from build123d import *

# Parameters (mm, degrees)
SKETCH1_W                    = 96
SKETCH1_H                    = 1
BASE_FLANGE1_DEPTH           = 329.72
EDGE_FLANGE1_STRIP_W         = 5.4732
EDGE_FLANGE1_STRIP_H         = 1
EDGE_FLANGE1_STRIP_CUT_DEPTH = 96
EDGE_FLANGE1_DEPTH           = 96
EDGE_FLANGE2_STRIP_W         = 5.4732
EDGE_FLANGE2_STRIP_H         = 1
EDGE_FLANGE2_STRIP_CUT_DEPTH = 96
EDGE_FLANGE2_DEPTH           = 96
EDGE_FLANGE3_STRIP_W         = 5.4732
EDGE_FLANGE3_STRIP_H         = 1
EDGE_FLANGE3_STRIP_CUT_DEPTH = 96
EDGE_FLANGE3_DEPTH           = 96
EDGE_FLANGE4_STRIP_W         = 5.4732
EDGE_FLANGE4_STRIP_H         = 1
EDGE_FLANGE4_STRIP_CUT_DEPTH = 96
EDGE_FLANGE4_DEPTH           = 96
CUT_EXTRUDE1_DEPTH           = 10
SKETCH23_R                   = 8
CUT_EXTRUDE4_DEPTH           = 10


# Sheet-metal steps are written as plain solids
with BuildPart() as part:
    # Sketch1 → Base-Flange1 (new body)
    with BuildSketch(Plane.XY):
        with Locations((48, -0.5)):
            Rectangle(SKETCH1_W, SKETCH1_H)
    extrude(amount=BASE_FLANGE1_DEPTH)

    # Edge-Flange1 strip (across the edge) → Edge-Flange1 strip cut (cut)
    with BuildSketch(Plane(origin=(0, 0, 329.72), x_dir=(0, 0, -1), z_dir=(1, 0, 0))):
        with Locations((-1, -0.5)):
            Rectangle(EDGE_FLANGE1_STRIP_W, EDGE_FLANGE1_STRIP_H)
    extrude(amount=EDGE_FLANGE1_STRIP_CUT_DEPTH, mode=Mode.SUBTRACT)

    # Edge-Flange1 section (across the edge) → Edge-Flange1 (add)
    with BuildSketch(Plane(origin=(0, 0, 329.72), x_dir=(0, 0, -1), z_dir=(1, 0, 0))):
        with BuildLine():
            Line((0, 0.7366), (0, 35))
            Line((0, 35), (1, 35))
            Line((1, 35), (1, 0.7366))
            ThreePointArc((1, 0.7366), (1.215745145, 0.215745145), (1.7366, 0))
            Line((1.7366, 0), (1.7366, -1))
            ThreePointArc((1.7366, -1), (0.508638364, -0.491361636), (0, 0.7366))
        make_face()
    extrude(amount=EDGE_FLANGE1_DEPTH)

    # Edge-Flange2 strip (across the edge) → Edge-Flange2 strip cut (cut)
    with BuildSketch(Plane.ZY.offset(-96)):
        with Locations((-1, -0.5)):
            Rectangle(EDGE_FLANGE2_STRIP_W, EDGE_FLANGE2_STRIP_H)
    extrude(amount=EDGE_FLANGE2_STRIP_CUT_DEPTH, mode=Mode.SUBTRACT)

    # Edge-Flange2 section (across the edge) → Edge-Flange2 (add)
    with BuildSketch(Plane.ZY.offset(-96)):
        with BuildLine():
            Line((0, 0.7366), (0, 35))
            Line((0, 35), (1, 35))
            Line((1, 35), (1, 0.7366))
            ThreePointArc((1, 0.7366), (1.215745145, 0.215745145), (1.7366, 0))
            Line((1.7366, 0), (1.7366, -1))
            ThreePointArc((1.7366, -1), (0.508638364, -0.491361636), (0, 0.7366))
        make_face()
    extrude(amount=EDGE_FLANGE2_DEPTH)

    # Edge-Flange3 strip (across the edge) → Edge-Flange3 strip cut (cut)
    with BuildSketch(Plane(origin=(0, 35, 328.72), x_dir=(0, -1, 0), z_dir=(1, 0, 0))):
        with Locations((-1, -0.5)):
            Rectangle(EDGE_FLANGE3_STRIP_W, EDGE_FLANGE3_STRIP_H)
    extrude(amount=EDGE_FLANGE3_STRIP_CUT_DEPTH, mode=Mode.SUBTRACT)

    # Edge-Flange3 section (across the edge) → Edge-Flange3 (add)
    with BuildSketch(Plane(origin=(0, 35, 328.72), x_dir=(0, -1, 0), z_dir=(1, 0, 0))):
        with BuildLine():
            Line((0, 0.7366), (0, 27))
            Line((0, 27), (1, 27))
            Line((1, 27), (1, 0.7366))
            ThreePointArc((1, 0.7366), (1.215745145, 0.215745145), (1.7366, 0))
            Line((1.7366, 0), (1.7366, -1))
            ThreePointArc((1.7366, -1), (0.508638364, -0.491361636), (0, 0.7366))
        make_face()
    extrude(amount=EDGE_FLANGE3_DEPTH)

    # Edge-Flange4 strip (across the edge) → Edge-Flange4 strip cut (cut)
    with BuildSketch(Plane(origin=(96, 35, 1), x_dir=(0, -1, 0), z_dir=(-1, 0, 0))):
        with Locations((-1, -0.5)):
            Rectangle(EDGE_FLANGE4_STRIP_W, EDGE_FLANGE4_STRIP_H)
    extrude(amount=EDGE_FLANGE4_STRIP_CUT_DEPTH, mode=Mode.SUBTRACT)

    # Edge-Flange4 section (across the edge) → Edge-Flange4 (add)
    with BuildSketch(Plane(origin=(96, 35, 1), x_dir=(0, -1, 0), z_dir=(-1, 0, 0))):
        with BuildLine():
            Line((0, 0.7366), (0, 27))
            Line((0, 27), (1, 27))
            Line((1, 27), (1, 0.7366))
            ThreePointArc((1, 0.7366), (1.215745145, 0.215745145), (1.7366, 0))
            Line((1.7366, 0), (1.7366, -1))
            ThreePointArc((1.7366, -1), (0.508638364, -0.491361636), (0, 0.7366))
        make_face()
    extrude(amount=EDGE_FLANGE4_DEPTH)

    # Sketch22 → Cut-Extrude1 (cut)
    with BuildSketch(Plane(origin=(0, 0, 0), x_dir=(1, 0, 0), z_dir=(0, 1, 0))):
        with BuildLine():
            Line((70, -214.9834), (70, -287.9834))
            ThreePointArc((70, -287.9834), (77, -294.9834), (84, -287.9834))
            Line((84, -287.9834), (84, -214.9834))
            ThreePointArc((84, -214.9834), (77, -207.9834), (70, -214.9834))
        make_face()
        with BuildLine():
            Line((70, -114.7366), (70, -41.7366))
            ThreePointArc((70, -41.7366), (77, -34.7366), (84, -41.7366))
            Line((84, -41.7366), (84, -114.7366))
            ThreePointArc((84, -114.7366), (77, -121.7366), (70, -114.7366))
        make_face()
    extrude(amount=-CUT_EXTRUDE1_DEPTH, mode=Mode.SUBTRACT)

    # Sketch23 → Cut-Extrude4 (cut)
    with BuildSketch(Plane(origin=(0, 0, 0), x_dir=(1, 0, 0), z_dir=(0, 1, 0))):
        with Locations(Location((25, -164.86, 0), (0, 0, 270))):
            Circle(SKETCH23_R)
    extrude(amount=-CUT_EXTRUDE4_DEPTH, mode=Mode.SUBTRACT)


solid = part.part
Input: part model. Units: mm. Frame: model coordinates. A direction names the side the tool comes from. Round coordinates to 2 decimals unless told otherwise and drop trailing zeros. Order: outer loops, then holes, each group sorted by start corner. A loop starts at its lowest first (then second) coordinate and runs counter-clockwise, first axis right, second up. Notation, with made-up numbers: (36.5, 7) - (46.5, 7) arc R22 ccw to (46.5, 26) - close; hole circle Ø9 at (60, 29.25). An arc over 180 degrees is marked (long way). Use a Markdown table: item, result.
1. Access query for faces 1 (the face through (47, 35, 315)), 2 (the face through (77.154, -0.493, 121.735)), 3 (the face through (47, 17, 328.72)). Directions: +Z, -Z, +X, -X, +Y, -Y. A direction counts if a zero-diameter tool reaches every point of the face in a straight line with its end or side. Return the directions, or none.
Evaluation:
| item | result |
|---|---|
| face 1 | +Z, -Z, +X, -X, +Y |
| face 2 | +Y, -Y |
| face 3 | +X, -X |
2. Section B-B on x = 77. Return the cut outline in (y, z), then the cut area to 3 significant figures.
Evaluation:
| item | result |
|---|---|
| outline | (-1, 1.74) arc R1.74 ccw to (0.74, 0) - (33.26, 0) arc R1.74 ccw to (35, 1.74) - (35, 28) - (34, 28) - (34, 1.74) arc R0.74 cw to (33.26, 1) - (0.74, 1) arc R0.74 cw to (0, 1.74) - (0, 34.74) - (-1, 34.74) - close; (-1, 121.74) - (0, 121.74) - (0, 207.98) - (-1, 207.98) - close; (-1, 294.98) - (0, 294.98) - (0, 327.98) arc R0.74 cw to (0.74, 328.72) - (33.26, 328.72) arc R0.74 cw to (34, 327.98) - (34, 301.72) - (35, 301.72) - (35, 327.98) arc R1.74 ccw to (33.26, 329.72) - (0.74, 329.72) arc R1.74 ccw to (-1, 327.98) - close |
| area | 278 mm^2 |
3. Section A-A on y = 13.5. Return the cut outline in (x, z).
Evaluation:
| item | result |
|---|---|
| outline | (0, 0) - (96, 0) - (96, 1) - (0, 1) - close; (0, 328.72) - (96, 328.72) - (96, 329.72) - (0, 329.72) - close |
4. Mould query, pull axis Y, two halves, no side actions, for faces 4 (the face through (49, 35, 15)), 5 (the face through (49, 34, 15)), 6 (the face through (49, 17, 0)), 7 (the face through (47, 0, 163)). Classes: +Y half, -Y half, draft (parallel to the pull), parting line (faces both ways), or undercut.
Evaluation:
| item | result |
|---|---|
| face 4 | +Y half |
| face 5 | undercut |
| face 6 | draft |
| face 7 | undercut |
5. Section C-C on z = 164.86. Return the cut outline in (x, y).
Evaluation:
| item | result |
|---|---|
| outline | (0, -1) - (17, -1) - (17, 0) - (0, 0) - close; (33, -1) - (96, -1) - (96, 0) - (33, 0) - close |
6. Section D-D on x = 25. Return the cut outline in (y, z), then the cut area to 3 significant figures.
Evaluation:
| item | result |
|---|---|
| outline | (-1, 1.74) arc R1.74 ccw to (0.74, 0) - (33.26, 0) arc R1.74 ccw to (35, 1.74) - (35, 28) - (34, 28) - (34, 1.74) arc R0.74 cw to (33.26, 1) - (0.74, 1) arc R0.74 cw to (0, 1.74) - (0, 156.86) - (-1, 156.86) - close; (-1, 172.86) - (0, 172.86) - (0, 327.98) arc R0.74 cw to (0.74, 328.72) - (33.26, 328.72) arc R0.74 cw to (34, 327.98) - (34, 301.72) - (35, 301.72) - (35, 327.98) arc R1.74 ccw to (33.26, 329.72) - (0.74, 329.72) arc R1.74 ccw to (-1, 327.98) - close |
| area | 436 mm^2 |
7. Material intervals for probe 1 along X at (y, z) = (-0.7, 164.86); probe 2 along Z at (x, y) = (50, 19.5); probe 3 along Y at (x, z) = (64.5, 304), sorted ascending.
Evaluation:
| item | result |
|---|---|
| probe 1 | 0 to 17, 33 to 96 |
| probe 2 | 0 to 1, 328.72 to 329.72 |
| probe 3 | -1 to 0, 34 to 35 |
8. First-contact query: pin 1 (9.5 mm diameter, centred on x = 25, z = 164.86, fed in from +Y); pin 2 (1.1 mm diameter, centred on x = 53, y = 34.5, fed in from +Z); pin 3 (0.5 mm diameter, centred on x = 51.5, y = 34.5, fed in from -Z); pin 4 (3 mm diameter, centred on x = 28.5, z = 75.5, fed in from +Y). Flat tips, straight axial feed; report the tip coordinate or a pass-through.
Evaluation:
| item | result |
|---|---|
| pin 1 | through |
| pin 2 | z = 329.58 |
| pin 3 | z = 0.31 |
| pin 4 | y = 0 |
